Design review of the part shown in the three views and the two pictorial views. Dimensions are in mm from the part's minimum x, y and z. A direction names the side the tool comes from. Coordinates: 2 decimals unless noted, no trailing zeros. Order: outer loops, then holes, each group sorted by start corner. A loop starts at its lowest first (then second) coordinate and runs counter-clockwise, first axis right, second up. Notation, with made-up numbers: (-33.75, -8) -> (1.25, -8) arc R11 cw to (1.25, -2) -> close; hole circle Ø1 at (-6.5, 69). An arc over 180 degrees is marked (long way). Answer as a JSON object with one key per item and string values. Group by question number.
1) Draft analysis for pull direction Z (two halves, no side actions). For the marked faces 1, 2 and 3, state which applies: +Z half, -Z half, draft (parallel to the pull), parting line (faces both ways), or undercut.
2) Add section A-A, the plane y = 3.5. Write out the cut boundary in (x, z), then the cut area to 3 significant figures.
3) Add section C-C, the plane x = 37.5. Write out the cut boundary in (y, z), then the cut area to 3 significant figures.
4) Wall thickness on L1, parallel to Z at x = 6, y = 2.5; L2, parallel to X at y = 5.5, z = 32; L3, parallel to Y at x = 12, z = 33: over which ranges is each line inside the solid? List them lowest first.
5) For pin 1 (16 mm diameter, centred on x = 32, z = 22, fed in from +Y); pin 2 (3 mm diameter, centred on y = 4.5, z = 24, fed in from -X), all flat-tipped, find the tip position at first contact; note any pin that passes through.
6) Add section D-D, the plane z = 10. Write out the cut boundary in (x, y).
7) Add section B-B, the plane z = 32.5. Write out the cut boundary in (x, y).
8) Machinability: for the marked faces 4 and 5, which of the approach directions +Z, -Z, +X, -X, +Y, -Y give a long, thin tool a straight path to every point of the face, cutting with its end or side? Answer none if there is none.
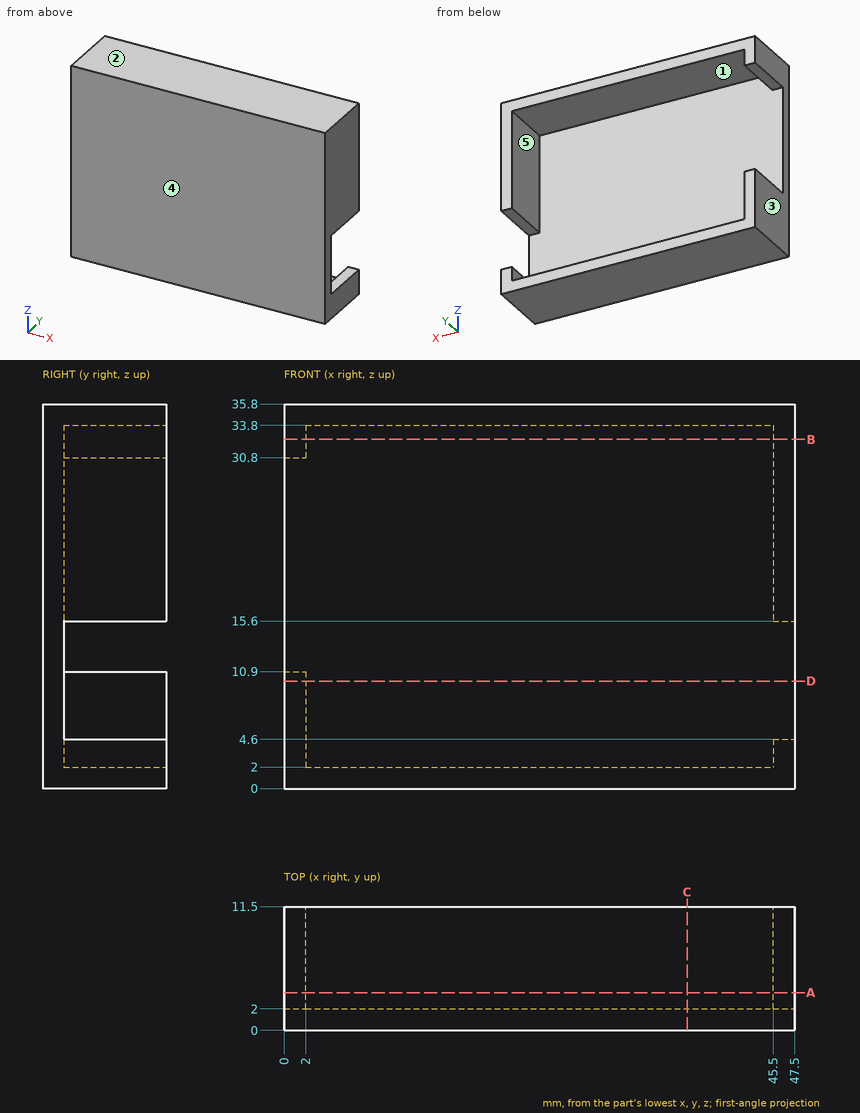
Output values:
{
 "1": {"face 1": "undercut", "face 2": "+Z half", "face 3": "draft"},
 "2": {"outline": "(0, 0) -> (47.5, 0) -> (47.5, 4.6) -> (45.5, 4.6) -> (45.5, 2) -> (2, 2) -> (2, 10.9) -> (0, 10.9) -> close; (0, 30.8) -> (2, 30.8) -> (2, 33.8) -> (45.5, 33.8) -> (45.5, 15.6) -> (47.5, 15.6) -> (47.5, 35.8) -> (0, 35.8) -> close", "area": "255 mm²"},
 "3": {"outline": "(0, 0) -> (11.5, 0) -> (11.5, 2) -> (2, 2) -> (2, 33.8) -> (11.5, 33.8) -> (11.5, 35.8) -> (0, 35.8) -> close", "area": "110 mm²"},
 "4": {"L1": "z = 0 to 2, 33.8 to 35.8", "L2": "x = 0 to 2, 45.5 to 47.5", "L3": "y = 0 to 2"},
 "5": {"pin 1": "stops at y = 2", "pin 2": "stops at x = 45.5"},
 "6": {"outline": "(0, 0) -> (47.5, 0) -> (47.5, 2) -> (2, 2) -> (2, 11.5) -> (0, 11.5) -> close"},
 "7": {"outline": "(0, 0) -> (47.5, 0) -> (47.5, 11.5) -> (45.5, 11.5) -> (45.5, 2) -> (2, 2) -> (2, 11.5) -> (0, 11.5) -> close"},
 "8": {"face 4": "+Z, -Z, +X, -X, -Y", "face 5": "+Y"}
}
